Work out the finished part from the listing and answer in its coordinate system (mm). A direction names the side the tool comes from. Give positions to 0.01 mm unless a question says otherwise; leave off trailing zeros. Loops run counter-clockwise (first coordinate to the right, second up) from the corner with the lowest first, then second, coordinate; pieces in that order, holes last. Notation, with made-up numbers: (2.5, 75.5) - (61.5, 75.5) arc R11 ccw to (61.5, 89.5) - close; hole circle Ø3 at (3.25, 36). An arc over 180 degrees is marked (long way). One line per item, written item: value.
from build123d import *

# Parameters (mm, degrees)
SKETCH_1_W           = 20
SKETCH_1_H           = 20
SKETCH_1_W_2         = 16
SKETCH_1_H_2         = 16
EXTRUDE_1_DEPTH      = 970
CUT_EXTRUDE_1_DEPTH  = 20
CUT_EXTRUDE_2_DEPTH  = 10
SKETCH_6_W           = 27.825743136
SKETCH_6_H           = 21.841712354
CUT_EXTRUDE_8_DEPTH  = 50
SKETCH_9_R           = 1
CUT_EXTRUDE_9_DEPTH  = 10
M4X0_7_3_D           = 3.3
M4X0_7_2_D           = 3.3
M4X0_7_7_D           = 3.3
M4X0_7_7_DEPTH       = 11.5
M4X0_7_7_TIP         = 0.991420021
M4X0_7_9_D           = 3.3
M4X0_7_9_DEPTH       = 11.5
M4X0_7_9_TIP         = 0.991420021
SKETCH_26_R          = 1
CUT_EXTRUDE_10_DEPTH = 10
M4X0_7_10_D          = 3.3
M4X0_7_10_DEPTH      = 11.5
M4X0_7_10_TIP        = 0.991420021


with BuildPart() as part:
    # ｽｹｯﾁ1 → ﾎﾞｽ - 押し出し1 (new body)
    with BuildSketch(Plane.XY):
        Rectangle(SKETCH_1_W, SKETCH_1_H)
        Rectangle(SKETCH_1_W_2, SKETCH_1_H_2, mode=Mode.SUBTRACT)
    extrude(amount=EXTRUDE_1_DEPTH)

    # ｽｹｯﾁ2 → ｶｯﾄ - 押し出し1 (cut)
    with BuildSketch(Plane(origin=(10, 0, 0), x_dir=(0, 0, -1), z_dir=(1, 0, 0))):
        with BuildLine():
            ThreePointArc((-45.75, 0), (-50, 4.25), (-54.25, 0))
            Line((-54.25, 0), (-50, 0))
            Line((-50, 0), (-45.75, 0))
        make_face()
        with BuildLine():
            Line((-50, 0), (-54.25, 0))
            ThreePointArc((-54.25, 0), (-50, -4.25), (-45.75, 0))
            Line((-45.75, 0), (-50, 0))
        make_face()
    extrude(amount=-CUT_EXTRUDE_1_DEPTH, mode=Mode.SUBTRACT)

    # ｽｹｯﾁ3 → ｶｯﾄ - 押し出し2 (cut)
    with BuildSketch(Plane(origin=(0, 10, 0), x_dir=(1, 0, 0), z_dir=(0, 1, 0))):
        with BuildLine():
            ThreePointArc((0, -649), (-1, -650), (0, -651))
            Line((0, -651), (0, -650))
            Line((0, -650), (0, -649))
        make_face()
        with BuildLine():
            Line((0, -650), (0, -651))
            ThreePointArc((0, -651), (0.707106781, -650.707106781), (1, -650))
            ThreePointArc((1, -650), (0.707106781, -649.292893219), (0, -649))
            Line((0, -649), (0, -650))
        make_face()
        with BuildLine():
            ThreePointArc((0, -669), (-1, -670), (0, -671))
            Line((0, -671), (0, -670))
            Line((0, -670), (0, -669))
        make_face()
        with BuildLine():
            Line((0, -670), (0, -671))
            ThreePointArc((0, -671), (0.707106781, -670.707106781), (1, -670))
            ThreePointArc((1, -670), (0.707106781, -669.292893219), (0, -669))
            Line((0, -669), (0, -670))
        make_face()
    extrude(amount=-CUT_EXTRUDE_2_DEPTH, mode=Mode.SUBTRACT)

    # ｽｹｯﾁ6 → ｶｯﾄ - 押し出し8 (cut)
    with BuildSketch(Plane.XY.offset(970)):
        Rectangle(SKETCH_6_W, SKETCH_6_H)
    extrude(amount=-CUT_EXTRUDE_8_DEPTH, mode=Mode.SUBTRACT)

    # ｽｹｯﾁ9 → ｶｯﾄ - 押し出し9 (cut)
    with BuildSketch(Plane(origin=(0, 10, 0), x_dir=(1, 0, 0), z_dir=(0, 1, 0))):
        with Locations((0, -30)):
            Circle(SKETCH_9_R)
        with Locations((0, -50)):
            Circle(SKETCH_9_R)
    extrude(amount=-CUT_EXTRUDE_9_DEPTH, mode=Mode.SUBTRACT)

    # M4x0.7 ねじ穴3 (through all)
    with Locations(Plane(origin=(0, 10, 111.21), x_dir=(1, 0, 0), z_dir=(0, 1, 0))):
        with Locations((0, 0), (0, -29)):
            Hole(M4X0_7_3_D / 2)

    # M4x0.7 ねじ穴2 (through all)
    with Locations(Plane(origin=(0, 10, 125.71), x_dir=(1, 0, 0), z_dir=(0, 1, 0))):
        with Locations((0, 0)):
            Hole(M4X0_7_2_D / 2)

    # M4x0.7 ねじ穴7
    with Locations(Plane(origin=(0, 10, 650), x_dir=(1, 0, 0), z_dir=(0, 1, 0))):
        with Locations((0, 0), (0, -20)):
            Hole(M4X0_7_7_D / 2, depth=M4X0_7_7_DEPTH)
            with Locations((0, 0, -(M4X0_7_7_DEPTH + M4X0_7_7_TIP / 2))):  # 118° drill point
                Cone(0, M4X0_7_7_D / 2, M4X0_7_7_TIP, mode=Mode.SUBTRACT)

    # M4x0.7 ねじ穴9
    with Locations(Plane(origin=(0, 10, 30), x_dir=(1, 0, 0), z_dir=(0, 1, 0))):
        with Locations((0, 0), (0, -20)):
            Hole(M4X0_7_9_D / 2, depth=M4X0_7_9_DEPTH)
            with Locations((0, 0, -(M4X0_7_9_DEPTH + M4X0_7_9_TIP / 2))):  # 118° drill point
                Cone(0, M4X0_7_9_D / 2, M4X0_7_9_TIP, mode=Mode.SUBTRACT)

    # ｽｹｯﾁ26 → ｶｯﾄ - 押し出し10 (cut)
    with BuildSketch(Plane.ZY.offset(10)):
        with Locations((40, 0)):
            Circle(SKETCH_26_R)
        with Locations((710, 0)):
            Circle(SKETCH_26_R)
        with Locations((730, 0)):
            Circle(SKETCH_26_R)
    extrude(amount=-CUT_EXTRUDE_10_DEPTH, mode=Mode.SUBTRACT)

    # M4x0.7 ねじ穴10
    with Locations(Plane(origin=(-10, 0, 730), x_dir=(0, 0, -1), z_dir=(-1, 0, 0))):
        with Locations((0, 0), (20, 0), (690, 0)):
            Hole(M4X0_7_10_D / 2, depth=M4X0_7_10_DEPTH)
            with Locations((0, 0, -(M4X0_7_10_DEPTH + M4X0_7_10_TIP / 2))):  # 118° drill point
                Cone(0, M4X0_7_10_D / 2, M4X0_7_10_TIP, mode=Mode.SUBTRACT)


solid = part.part
1. For faces 1 (the flat face through (-9, 0, 920)), 2 (the flat face through (0, -8, 454)), determine the directions among +Z, -Z, +X, -X, +Y, -Y from which every point of the face is accessible in a straight line to the end or side of a thin tool.
Output:
face 1: +Z, +X, -X, +Y, -Y
face 2: +Z, -Z
2. Section B-B (z = 458) is taken. Write down the section's boundary in (x, y), and give its area (3 significant figures).
Output:
outline: (-10, -10) - (10, -10) - (10, 10) - (-10, 10) - close; hole (-8, -8) - (8, -8) - (8, 8) - (-8, 8) - close
area: 144 mm²
3. Find the intervals of material crossed by line 1 along Z through (x, y) = (0, -9.55); line 2 along X through (y, z) = (-5.5, 853), in increasing order.
Output:
line 1: z = 0 to 109.56, 112.86 to 124.06, 127.36 to 138.56, 141.86 to 920
line 2: x = -10 to -8, 8 to 10
4. The mould has two halves that part along X. Classify faces 3 (the flat face through (-10, 0, 454)), 4 (the flat face through (0, -10, 454)), 5 (the flat face through (0, 8, 454)): released by +X, released by -X, zero draft, split by the parting line, or undercut.
Output:
face 3: released by -X
face 4: zero draft
face 5: undercut
5. Section A-A (x = 5) is taken. Write down the section's boundary in (y, z).
Output:
outline: (-10, 0) - (-8, 0) - (-8, 920) - (-10, 920) - close; (8, 0) - (10, 0) - (10, 920) - (8, 920) - close
6. Flat-ended cylindrical pins translate along their axes: pin 1 Ø4.5 at (x, z) = (0, 111.21) entering from -Y; pin 2 Ø3 at (x, z) = (0, 30) entering from +Y. Find the tip coordinate at first contact, or state that the pin passes through.
Output:
pin 1: stops at y = -10
pin 2: stops at y = -8
